Source: CAD feature listing. Evaluate the final solid. Frame: model axes, mm. A direction names the side the tool comes from. Round coordinates to 2 decimals unless told otherwise and drop trailing zeros. Write each loop counter-clockwise with the first axis right and the second up, starting at its lowest first coordinate (ties: lowest second). Pieces come first, ordered by that corner, then holes.
from build123d import *

# Parameters (mm, degrees)
F0_R      = 25.4
F1_DEPTH  = 19.05
F2_R      = 1.5875
F3_DEPTH  = 44.45
F4_R      = 5.08
F5_R      = 22.225
F6_DEPTH  = 19.05
F7_R      = 25.4
F8_DEPTH  = 19.05
F10_R     = 6.35
F11_DEPTH = 57.1510001


# Not quite as in the source:
# - a fillet or chamfer that OpenCascade refuses, or shapes differently, is made with other operations: its cross-section is extruded or revolved along the edge and cut away or added


with BuildPart() as f1:
    # F0 (on Front) → F1 (new body)
    with BuildSketch(Plane.XZ):
        Circle(F0_R)
    extrude(amount=F1_DEPTH)

    # F2 (on face) → F3 (cut)
    with BuildSketch(Plane(origin=(0, 0, 0), x_dir=(-1, 0, 0), z_dir=(0, 1, 0))):
        with Locations((0, 16.1551559669)):
            Circle(F2_R)
        with Locations((16.5286865403, 0)):
            Circle(F2_R)
        with Locations((0, -18.7698644697)):
            Circle(F2_R)
        with Locations((-17.8360380362, 0)):
            Circle(F2_R)
    extrude(amount=-F3_DEPTH, mode=Mode.SUBTRACT)

    # F4
    f4_edges = [f1.edges().sort_by_distance(p)[0] for p in [
        (-25.4, 0, 0),
        (-25.4, -19.05, 0),
    ]]
    fillet(f4_edges, radius=F4_R)

    # F5 (on Front) → F6 (join)
    with BuildSketch(Plane.XZ):
        Circle(F5_R)
    extrude(amount=-F6_DEPTH)

    # F7 (on face) → F8 (join)
    with BuildSketch(Plane(origin=(0, 19.05, 0), x_dir=(-1, 0, 0), z_dir=(0, 1, 0))):
        Circle(F7_R)
    extrude(amount=F8_DEPTH)

    # F9: fillet of radius 5.08 on 2 edges, made by hand

    # F9_s1 → F9_t2 (revolve, cut)
    with BuildSketch(Plane.XY):
        with BuildLine():
            ThreePointArc((-25.4, 33.02), (-23.9121024484, 36.6121024484), (-20.32, 38.1))
            Line((-20.32, 38.1), (-25.4, 38.1))
            Line((-25.4, 38.1), (-25.4, 33.02))
        make_face()
    revolve(axis=Axis((0, 38.1, 0), (0, 1, 0)), mode=Mode.SUBTRACT)

    # F9_s3 → F9_t4 (revolve, cut)
    with BuildSketch(Plane.XY):
        with BuildLine():
            ThreePointArc((-25.4, 23.7592860393), (-24.5321134838, 20.9194797079), (-22.225, 19.05))
            Line((-22.225, 19.05), (-25.4, 19.05))
            Line((-25.4, 19.05), (-25.4, 23.7592860393))
        make_face()
    revolve(axis=Axis((0, 19.05, 0), (0, 1, 0)), mode=Mode.SUBTRACT)

    # F10 (on face) → F11 (cut, through all)
    with BuildSketch(Plane(origin=(0, 38.1, 0), x_dir=(-1, 0, 0), z_dir=(0, 1, 0))):
        Circle(F10_R)
    extrude(amount=-F11_DEPTH, mode=Mode.SUBTRACT)


solid = f1.part
1) Material intervals for line 1 (Z direction, x = 0, y = -14.5); line 2 (X direction, y = 34, z = 5); line 3 (Z direction, x = -5.5, y = 17), sorted ascending.
Taken from the geometry:
line 1: z = -25.37 to -20.36, -17.18 to -6.35, 6.35 to 14.57, 17.74 to 25.37
line 2: x = -24.81 to -3.91, 3.91 to 24.81
line 3: z = -21.53 to -3.17, 3.17 to 21.53
2) Contact query for flat-ended pins moving along their axis: P1, Ø4, axis at x = -3.5, y = 4, coming from the +Z side; P2, Ø1, axis at x = -16, z = 0.5, coming from the -Y side; P3, Ø6, axis at x = -18.5, y = 28.5, coming from the -Z side; P4, Ø11.5, axis at x = 0, z = 0, coming from the -Y side (3 decimals). Output: stop coordinate, or through.
Taken from the geometry:
P1: stops at z = 22.17
P2: stops at y = 0
P3: stops at z = -20.12
P4: passes through
3) Section query C-C on y = 23. Return the cut outline in (x, z).
Taken from the geometry:
outline: circle Ø50.69 at (0, 0); hole circle Ø12.7 at (0, 0)
4) Section query A-A on y = -6.5. State how many separate pieces and enclosed holes the cut face has, then the cut area to 3 significant figures.
Taken from the geometry:
separate pieces: 1
enclosed holes: 5
area: 1,870 mm2
5) Pull-direction query (Z, two-part tool) for faces 1 (the face through (19.42, -9.39, 0.07)), 2 (the face through (-5, -19.05, 5)), 3 (the face through (-5.506, -9.463, -24.796)); classes: released by +Z, released by -Z, zero draft, split by the parting line, or undercut.
Taken from the geometry:
face 1: undercut
face 2: zero draft
face 3: split by the parting line
6) Reachability of faces 4 (the face through (21.199, 9.392, 6.676)), 5 (the face through (5, 38.1, 5)), 6 (the face through (0, 0, -19)) from +Z, -Z, +X, -X, +Y, -Y: full face, straight path, thin tool, end or side. Return the list, or none.
Taken from the geometry:
face 4: none
face 5: +Z, -Z, +X, -X, +Y
face 6: -Y
7) Section query B-B on y = 7. Return the cut outline in (x, z) (3 decimals).
Taken from the geometry:
outline: circle Ø44.45 at (0, 0); hole circle Ø12.7 at (0, 0)
